```python
from build123d import *

# Parameters (mm, degrees)
SKETCH1_W               = 11.811
SKETCH1_H               = 45.98924
BOSS_EXTRUDE1_DEPTH     = 9.652
FILLET5_R               = 4.826
SKETCH2_W               = 7.62
SKETCH2_H               = 22.352
CUT_EXTRUDE1_DEPTH      = 7.62
CUT_EXTRUDE2_DEPTH      = 49.452771033
CUT_EXTRUDE2_DEPTH_BACK = 49.452771033
SKETCH3_R               = 2.20345
FILLET4_R               = 4.826
FILLET6_R               = 10.16
CUT_EXTRUDE3_DEPTH      = 49.452771033
CUT_EXTRUDE4_DEPTH      = 7.62
BOSS_EXTRUDE2_DEPTH     = 7.62


with BuildPart() as part:
    # Sketch1 → Boss-Extrude1 (new body)
    with BuildSketch(Plane.XY):
        with Locations((5.9055, 22.99462)):
            Rectangle(SKETCH1_W, SKETCH1_H)
    extrude(amount=BOSS_EXTRUDE1_DEPTH)

    # Fillet5
    fillet5_edges = [part.edges().sort_by_distance(p)[0] for p in [
        (5.9055, 45.98924, 0),
    ]]
    fillet(fillet5_edges, radius=FILLET5_R)

    # Sketch2 → Cut-Extrude1 (cut)
    with BuildSketch(Plane(origin=(0, 0, 0), x_dir=(-1, 0, 0), z_dir=(0, 0, -1))):
        with Locations((-5.9055, 34.81324)):
            Rectangle(SKETCH2_W, SKETCH2_H)
    extrude(amount=-CUT_EXTRUDE1_DEPTH, mode=Mode.SUBTRACT)

    # Sketch3 → Cut-Extrude2 (cut, two sides: drawn at the far end of the back side and taken through both)
    with BuildSketch(Plane.ZY.offset(-CUT_EXTRUDE2_DEPTH_BACK)):
        with Locations((4.4323, 26.82494)):
            Circle(SKETCH3_R)
    extrude(amount=CUT_EXTRUDE2_DEPTH + CUT_EXTRUDE2_DEPTH_BACK, mode=Mode.SUBTRACT)

    # Fillet4
    # the kernel refuses this fillet: 4.826 mm, written as the material it takes off along each edge
    with BuildSketch(Plane(origin=(23.876, 45.98924, 9.652), x_dir=(0, 0, -1), z_dir=(-1, 0, 0))) as fillet4_piece_1:
        with BuildLine():
            CenterArc((FILLET4_R, FILLET4_R), FILLET4_R, 180, 90)
            Line((0, FILLET4_R), (0, 0))
            Line((0, 0), (FILLET4_R, 0))
        make_face()
    extrude(amount=35.941, mode=Mode.SUBTRACT)

    # Fillet6
    # the kernel refuses this fillet: 10.16 mm, written as the material it takes off along each edge
    with BuildSketch(Plane(origin=(-25.368230131, 0, 9.652), x_dir=(0, 1, 0), z_dir=(1, 0, 0))) as fillet6_piece_1:
        with BuildLine():
            CenterArc((10.147292053, -10.16), FILLET6_R, 90, 87.134016017)
            Line((0, -9.652), (-0.202945841, -9.64184))
            ThreePointArc((-0.202945841, -9.64184), (-0.2032, -4.826), (-0.2032, 0))
            Line((-0.2032, 0), (0, 0.2032))
            Line((0, 0.2032), (10.147292053, 0.2032))
            Line((10.147292053, 0.2032), (10.147292053, 0))
        make_face()
    extrude(amount=62.547460263, mode=Mode.SUBTRACT)

    # Sketch4 → Cut-Extrude3 (cut, through all)
    with BuildSketch(Plane(origin=(11.811, 0, 0), x_dir=(0, 0, -1), z_dir=(1, 0, 0))):
        Polygon((-9.652, 32.118813088), (-7.62, 36.34994), (0, 36.34994), (0, 45.98924), (-9.652, 45.98924), align=None)
    extrude(amount=-CUT_EXTRUDE3_DEPTH, mode=Mode.SUBTRACT)

    # Sketch5 → Cut-Extrude4 (cut)
    with BuildSketch(Plane.ZY.offset(-9.7155)):
        Polygon((0, 21.160076085), (5.158068358, 23.63724), (0, 23.63724), align=None)
    extrude(amount=CUT_EXTRUDE4_DEPTH, mode=Mode.SUBTRACT)

    # Sketch5<3> → Boss-Extrude2 (add)
    with BuildSketch(Plane.ZY.offset(-9.7155)):
        with BuildLine():
            Line((5.812301369, 23.951435604), (5.158068358, 23.63724))
            Line((5.158068358, 23.63724), (7.62, 23.63724))
            Line((7.62, 23.63724), (7.62, 26.82494))
            ThreePointArc((7.62, 26.82494), (7.130490287, 25.127530072), (5.812301369, 23.951435604))
        make_face()
    extrude(amount=BOSS_EXTRUDE2_DEPTH)


solid = part.part
```
Work out the finished part from the listing and answer in its coordinate system (mm). A direction names the side the tool comes from. Coordinates: 2 decimals unless noted, no trailing zeros. Write each loop counter-clockwise with the first axis right and the second up, starting at its lowest first coordinate (ties: lowest second). Pieces come first, ordered by that corner, then holes.
Q1. A cutting plane is placed at D-D, the plane x = 2.5. Give the vertices of the cut face in (y, z).
Q2. A cutting plane is placed at C-C, the plane x = 1. Give the vertices of the cut face in (y, z).
Q3. Which of the six approach directions +Z, -Z, +X, -X, +Y, -Y give full straight-line access (tool end or side, diameter ignored) to faces 1 (the face through (2.096, 30, 4)), 2 (the face through (1.06, 29.01, 4.15))?
Q4. Find the intervals of material crossed by line 1 (X direction, y = 29.5, z = 4); line 2 (Y direction, x = 11.25, z = 4.5); line 3 (Y direction, x = 10.5, z = 3), in increasing order.
Q5. This flat-tipped pin is pushed along its axis until it touches: pin 1 Ø2.5 at (y, z) = (26.5, 4.5) entering from +X. Where does it stop, or does it pass through?
Q6. Determine the mould class of faces 3 (the face through (1, 36.35, 4)), 4 (the face through (5.959, 25.149, 7.144)), 5 (the face through (0, 18, 5)) for opening direction X: released by +X, released by -X, zero draft, split by the parting line, or undercut.
Q7. A cutting plane is placed at B-B, the plane z = 4. Give the vertices of the cut face in (x, y), then the cut area to 3 significant figures.
Q8. A cutting plane is placed at A-A, the plane y = 27.5. Give the vertices of the cut face in (x, z).
Findings below:
1. outline: (0, 0) - (21.16, 0) - (23.95, 5.81) arc R3.19 cw to (26.82, 7.62) - (36.35, 7.62) - (32.12, 9.65) - (10.15, 9.65) arc R10.16 ccw to start
2. outline: (0, 0) - (36.35, 0) - (36.35, 7.62) - (32.12, 9.65) - (10.15, 9.65) arc R10.16 ccw to start; hole circle Ø4.41 at (26.82, 4.43)
3. face 1: -Z, +Y
3. face 2: +X, -X
4. line 1: x = 0 to 2.1, 9.72 to 11.81
4. line 2: y = 1.31 to 24.62, 29.03 to 36.35
4. line 3: y = 0.61 to 25.15, 28.5 to 36.35
5. pin 1: passes through
6. face 3: zero draft
6. face 4: undercut
6. face 5: released by -X
7. outline: (0, 1.04) - (11.81, 1.04) - (11.81, 24.66) - (9.72, 24.66) - (9.72, 23.08) - (2.1, 23.08) - (2.1, 24.66) - (0, 24.66) - close; (0, 28.99) - (2.1, 28.99) - (2.1, 36.35) - (0, 36.35) - close; (9.72, 28.99) - (11.81, 28.99) - (11.81, 36.35) - (9.72, 36.35) - close
7. area: 298 mm2
8. outline: (0, 0) - (2.1, 0) - (2.1, 2.33) - (0, 2.33) - close; (0, 6.53) - (2.1, 6.53) - (2.1, 7.62) - (9.72, 7.62) - (9.72, 6.53) - (11.81, 6.53) - (11.81, 9.65) - (0, 9.65) - close; (9.72, 0) - (11.81, 0) - (11.81, 2.33) - (9.72, 2.33) - close
